Could you check a few things on this drawing? It's one solid part, dimensions in mm from its lowest x, y, z. Round coordinates to 2 decimals unless told otherwise and drop trailing zeros. Write each loop counter-clockwise with the first axis right and the second up, starting at its lowest first coordinate (ties: lowest second). Pieces come first, ordered by that corner, then holes. Notation, with made-up numbers: (-3, -21) -> (27, -21) arc R25 cw to (27, 8) -> close; hole circle Ø9 at (7.25, 87). An arc over 180 degrees is marked (long way). Answer in a Markdown table with one row per item. Add a question column.
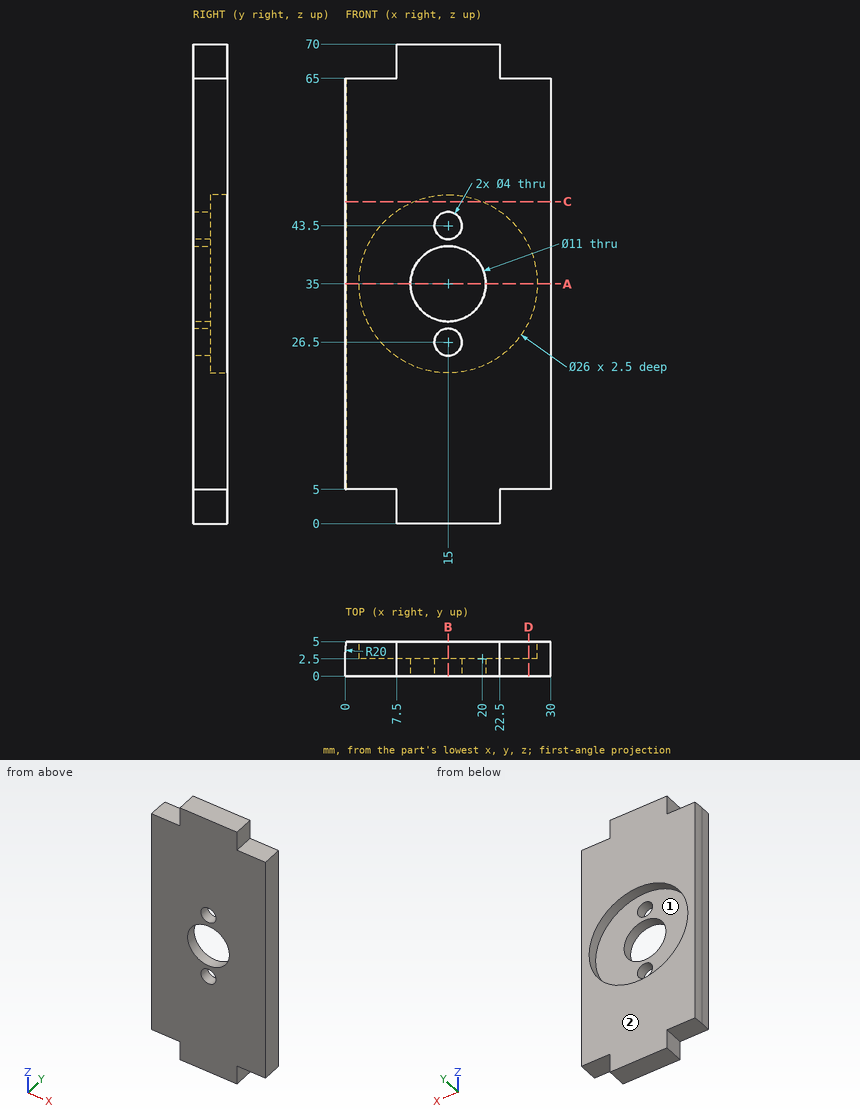
Item 1: I need wall thicknesses on line 1 along X through (y, z) = (3.1, 35); line 2 along X through (y, z) = (0.5, 26.5); line 3 along Y through (x, z) = (26.75, 32.5). Which ranges of each line are inside material? Lowest first, please. Write a range as from..to.
Item 2: If we mould it in two halves opening along X, with no side actions, what happens to the marked faces 1 and 2? For each: pulls with the +X half, pulls with the -X half, needs draft (parallel to the pull), parting line crosses it, or undercut.
Item 3: If we section it at D-D on x = 26.75: Please give me the cut outline in (y, z).
Item 4: If we section it at B-B on x = 15: Please give me the cut outline in (y, z).
Item 5: If we section it at A-A on z = 35: Please give me the cut outline in (x, y), then the cut area to 3 significant figures.
Item 6: For P1, Ø1.5, axis at y = 3.5, z = 3.5, coming from the -X side; P2, Ø17.5, axis at x = 15, z = 35, coming from the +Y side; P3, Ø1.5, axis at x = 27, y = 1.5, coming from the -Z side, each with a flat end and sliding along its axis, tell me the tip position at first contact or that it passes through.
Item 7: If we section it at C-C on z = 47: Please give me the cut outline in (x, y).
Results list:
| question | item | result |
|---|---|---|
| 1 | line 1 | 0.01..2, 28..30 |
| 1 | line 2 | 0..13, 17..30 |
| 1 | line 3 | 0..2.5 |
| 2 | face 1 | undercut |
| 2 | face 2 | needs draft |
| 3 | outline | (0, 5) -> (5, 5) -> (5, 29.44) -> (2.5, 29.44) -> (2.5, 40.56) -> (5, 40.56) -> (5, 65) -> (0, 65) -> close |
| 4 | outline | (0, 0) -> (5, 0) -> (5, 22) -> (2.5, 22) -> (2.5, 24.5) -> (0, 24.5) -> close; (0, 28.5) -> (2.5, 28.5) -> (2.5, 29.5) -> (0, 29.5) -> close; (0, 40.5) -> (2.5, 40.5) -> (2.5, 41.5) -> (0, 41.5) -> close; (0, 45.5) -> (2.5, 45.5) -> (2.5, 48) -> (5, 48) -> (5, 70) -> (0, 70) -> close |
| 5 | outline | (0, 0) -> (9.5, 0) -> (9.5, 2.5) -> (2, 2.5) -> (2, 5) -> (0.16, 5) arc R20 ccw to (0, 2.5) -> close; (20.5, 0) -> (30, 0) -> (30, 5) -> (28, 5) -> (28, 2.5) -> (20.5, 2.5) -> close |
| 5 | area | 57.4 mm² |
| 6 | P1 | x = 7.5 |
| 6 | P2 | y = 2.5 |
| 6 | P3 | z = 5 |
| 7 | outline | (0, 0) -> (30, 0) -> (30, 5) -> (20, 5) -> (20, 2.5) -> (10, 2.5) -> (10, 5) -> (0.16, 5) arc R20 ccw to (0, 2.5) -> close |
